from build123d import *

# Parameters (mm, degrees)
SKETCH1_W           = 85
SKETCH1_H           = 70
SKETCH1_R           = 1.375
SKETCH1_R_2         = 2
SKETCH1_R_3         = 4.125
SKETCH1_W_2         = 2.231847436
SKETCH1_H_2         = 6.309819942
SKETCH1_R_4         = 1.875
SKETCH1_R_5         = 3
BOSS_EXTRUDE4_DEPTH = 10
SKETCH1_7_R         = 4.5
CUT_EXTRUDE2_DEPTH  = 6
CUT_EXTRUDE6_DEPTH  = 6
SKETCH1_11_R        = 4.5
SKETCH1_11_R_2      = 3
CUT_EXTRUDE10_DEPTH = 8
SKETCH5_W           = 2.231847436
SKETCH5_H           = 6.309819942
BOSS_EXTRUDE5_DEPTH = 4


with BuildPart() as part:
    # Sketch1 → Boss-Extrude4 (new body)
    with BuildSketch(Plane(origin=(0, 0, 0), x_dir=(1, 0, 0), z_dir=(0, 1, 0))):
        Rectangle(SKETCH1_W, SKETCH1_H)
        with Locations((-27.5, -24.60667729)):
            Circle(SKETCH1_R, mode=Mode.SUBTRACT)
        with Locations((9.474989645, -16.722600152)):
            Circle(SKETCH1_R_2, mode=Mode.SUBTRACT)
        with Locations((22.5, -24.60667729)):
            Circle(SKETCH1_R, mode=Mode.SUBTRACT)
        with Locations((-15.52, 1)):
            Circle(SKETCH1_R_3, mode=Mode.SUBTRACT)
        with Locations((-8.615923718, 1)):
            Rectangle(SKETCH1_W_2, SKETCH1_H_2, mode=Mode.SUBTRACT)
        with Locations((-27.5, 25)):
            Circle(SKETCH1_R, mode=Mode.SUBTRACT)
        with Locations((9.330885495, 18.664687396)):
            Circle(SKETCH1_R_4, mode=Mode.SUBTRACT)
        with Locations((22.5, 25)):
            Circle(SKETCH1_R, mode=Mode.SUBTRACT)
        with Locations((16.478339488, 0.999882702)):
            Circle(SKETCH1_R_5, mode=Mode.SUBTRACT)
    extrude(amount=BOSS_EXTRUDE4_DEPTH)

    # Sketch1_7 → Cut-Extrude2 (cut)
    with BuildSketch(Plane(origin=(0, 0, 0), x_dir=(1, 0, 0), z_dir=(0, 1, 0))):
        with Locations((16.478339488, 0.999882702)):
            Circle(SKETCH1_7_R)
    extrude(amount=CUT_EXTRUDE2_DEPTH, mode=Mode.SUBTRACT)

    # Sketch1_9 → Cut-Extrude6 (cut)
    with BuildSketch(Plane(origin=(0, 0, 0), x_dir=(1, 0, 0), z_dir=(0, 1, 0))):
        with BuildLine():
            Line((12.955885495, 18.664687396), (12.955885495, 14.773048154))
            ThreePointArc((12.955885495, 14.773048154), (23.699805173, 1.074384413), (13.099989645, -12.736086581))
            Line((13.099989645, -12.736086581), (13.099989645, -16.722600152))
            ThreePointArc((13.099989645, -16.722600152), (9.474989645, -20.347600152), (5.849989645, -16.722600152))
            Line((5.849989645, -16.722600152), (5.849989645, -12.722879596))
            ThreePointArc((5.849989645, -12.722879596), (0.820287137, -10.238442268), (-2.854756169, -6))
            Line((-2.854756169, -6), (-7.5, -6))
            Line((-7.5, -6), (-7.5, 8))
            Line((-7.5, 8), (-2.854756169, 8))
            ThreePointArc((-2.854756169, 8), (0.761316141, 12.192649571), (5.705885495, 14.683738346))
            Line((5.705885495, 14.683738346), (5.705885495, 18.664687396))
            ThreePointArc((5.705885495, 18.664687396), (9.330885495, 22.289687396), (12.955885495, 18.664687396))
        make_face()
    extrude(amount=CUT_EXTRUDE6_DEPTH, mode=Mode.SUBTRACT)

    # Sketch1_11 → Cut-Extrude10 (cut)
    with BuildSketch(Plane(origin=(0, 0, 0), x_dir=(1, 0, 0), z_dir=(0, 1, 0))):
        with Locations((16.478339488, 0.999882702)):
            Circle(SKETCH1_11_R)
        with Locations((16.478339488, 0.999882702)):
            Circle(SKETCH1_11_R_2, mode=Mode.SUBTRACT)
    extrude(amount=CUT_EXTRUDE10_DEPTH, mode=Mode.SUBTRACT)

    # Sketch5 → Boss-Extrude5 (add)
    with BuildSketch(Plane(origin=(0, 10, 0), x_dir=(1, 0, 0), z_dir=(0, 1, 0))):
        with Locations((-8.615923718, 1)):
            Rectangle(SKETCH5_W, SKETCH5_H)
    extrude(amount=-BOSS_EXTRUDE5_DEPTH)


solid = part.part
Design review of the part built by this model. Coordinates are the model's own, in mm. A direction names the side the tool comes from. Give positions to 0.01 mm unless a question says otherwise; leave off trailing zeros. Write each loop counter-clockwise with the first axis right and the second up, starting at its lowest first coordinate (ties: lowest second). Pieces come first, ordered by that corner, then holes. Notation, with made-up numbers: M -3,63.25 L 42,63.25 A18 ccw 42,71.25 Z; hole C 77,-23 d1. An arc over 180 degrees is marked long. Return JSON: item names as keys, results as strings. Group by question number.
Item 1: Take a section at C-C (x = -15.52). Give the boundary of the cut face in (y, z) (3 decimals).
Item 2: Take a section at B-B (x = -27.5). Give the boundary of the cut face in (y, z) (3 decimals), plus the area to 3 significant figures.
Item 3: Take a section at A-A (z = -25). Give the boundary of the cut face in (x, y) (3 decimals), plus the area to 3 significant figures.
Item 4: Wall thickness on line 1 along X through (y, z) = (7.5, -25) (3 decimals); line 2 along X through (y, z) = (2.75, 16.5); line 3 along Z through (x, y) = (-28.5, 4): over which ranges is each line inside the solid? List them lowest first.
Item 5: Take a section at D-D (y = 2). Give the boundary of the cut face in (x, z) (3 decimals), plus the area to 3 significant figures.
Item 6: Clearance check with a flat-ended pin moving along its axis: pin 1 Ø2 at (x, z) = (-27.5, -25) entering from -Y. State where the tip first meets the part, or that it passes through.
Item 7: The part is to be moulded in two halves that separate along X. For faces 3 (the flat face through (-42.5, 5, 0)), 4 (the flat face through (15, 8, 2)), 5 (the flat face through (-1, 5, 35)), 6 (the cylindrical face through (19.25, 8.99, 0.15)), say which applies: pulls with the +X half, pulls with the -X half, needs draft (parallel to the pull), parting line crosses it, or undercut.
Item 8: Tool access review of faces 1 (the cylindrical face through (0.7, 2.958, -12.144)), 2 (the cylindrical face through (21.487, 4.93, -25.929)): name each direction out of +Z, -Z, +X, -X, +Y, -Y from which nothing blocks a thin tool from reaching the whole face with its end or side.
Return value:
{
 "1": {"outline": "M 0,-35 L 10,-35 L 10,-5.125 L 0,-5.125 Z; M 0,3.125 L 10,3.125 L 10,35 L 0,35 Z"},
 "2": {"outline": "M 0,-35 L 10,-35 L 10,-26.375 L 0,-26.375 Z; M 0,-23.625 L 10,-23.625 L 10,23.232 L 0,23.232 Z; M 0,25.982 L 10,25.982 L 10,35 L 0,35 Z", "area": "645 mm2"},
 "3": {"outline": "M -42.5,0 L -28.875,0 L -28.875,10 L -42.5,10 Z; M -26.125,0 L 21.125,0 L 21.125,10 L -26.125,10 Z; M 23.875,0 L 42.5,0 L 42.5,10 L 23.875,10 Z", "area": "795 mm2"},
 "4": {"line 1": "x = -42.5 to -28.875, -26.125 to 21.125, 23.875 to 42.5", "line 2": "x = -42.5 to 5.85, 13.1 to 42.5", "line 3": "z = -35 to -25.94, -24.06 to 23.66, 25.55 to 35"},
 "5": {"outline": "M -42.5,-35 L 42.5,-35 L 42.5,35 L -42.5,35 Z; hole C -27.5,-25 d2.75; hole C -27.5,24.607 d2.75; hole C -15.52,-1 d8.25; hole M -9.732,-4.155 L -7.5,-4.155 L -7.5,-8 L -2.855,-8 A14.2 ccw 5.706,-14.684 L 5.706,-18.665 A3.625 ccw 12.956,-18.665 L 12.956,-14.773 A14.2 ccw 13.1,12.736 L 13.1,16.723 A3.625 ccw 5.85,16.723 L 5.85,12.723 A14.2 ccw -2.855,6 L -7.5,6 L -7.5,2.155 L -9.732,2.155 Z; hole C 22.5,-25 d2.75; hole C 22.5,24.607 d2.75", "area": "5,080 mm2"},
 "6": {"pin 1": "passes through"},
 "7": {"face 3": "pulls with the -X half", "face 4": "undercut", "face 5": "needs draft", "face 6": "undercut"},
 "8": {"face 1": "-Y", "face 2": "+Y, -Y"}
}
